The listing builds one solid part. Answer for the finished solid, in the listing's coordinates (mm). Face numbers are marked on the shaded views. A direction names the side the tool comes from. Round coordinates to 2 decimals unless told otherwise and drop trailing zeros. Write each loop counter-clockwise with the first axis right and the second up, starting at its lowest first coordinate (ties: lowest second). Pieces come first, ordered by that corner, then holes. Notation, with made-up numbers: (28.5, -34.5) -> (56.5, -34.5) arc R17 cw to (56.5, -24.5) -> close; hole circle Ø2 at (1.5, 58.25). An arc over 180 degrees is marked (long way). Write each question's results on one line, items separated by ' | '. Start each with the question number.
```python
from build123d import *

# Parameters (mm, degrees)
F0_W     = 342.899989
F0_H     = 117.098217
F0_R     = 2.45745
F1_DEPTH = 19.05


with BuildPart() as f1:
    # F0 (on Top) → F1 (new body)
    with BuildSketch(Plane.XY):
        with Locations((199.415946, 93.865183)):
            Rectangle(F0_W, F0_H)
        with Locations((40.665952, 44.841074)):
            Circle(F0_R, mode=Mode.SUBTRACT)
        with Locations((120.040969, 57.604564)):
            Circle(F0_R, mode=Mode.SUBTRACT)
        with Locations((50.190963, 76.591074)):
            Circle(F0_R, mode=Mode.SUBTRACT)
        with Locations((149.674294, 76.591074)):
            Circle(F0_R, mode=Mode.SUBTRACT)
        with Locations((199.41597, 41.793069)):
            Circle(F0_R, mode=Mode.SUBTRACT)
        with Locations((278.79097, 57.604569)):
            Circle(F0_R, mode=Mode.SUBTRACT)
        with Locations((358.165952, 44.841074)):
            Circle(F0_R, mode=Mode.SUBTRACT)
        with Locations((249.157646, 76.591074)):
            Circle(F0_R, mode=Mode.SUBTRACT)
        with Locations((348.640962, 76.591074)):
            Circle(F0_R, mode=Mode.SUBTRACT)
        with Locations((50.190963, 105.166074)):
            Circle(F0_R, mode=Mode.SUBTRACT)
        with Locations((50.190963, 133.741074)):
            Circle(F0_R, mode=Mode.SUBTRACT)
        with Locations((34.315952, 146.064291)):
            Circle(F0_R, mode=Mode.SUBTRACT)
        with Locations((149.674294, 133.741081)):
            Circle(F0_R, mode=Mode.SUBTRACT)
        with BuildLine():
            ThreePointArc((66.451155, 86.116074), (59.715963, 86.116074), (59.715963, 92.851266))
            Line((59.715963, 92.851266), (59.715963, 117.480882))
            ThreePointArc((59.715963, 117.480882), (59.715963, 124.216074), (66.451155, 124.216074))
            Line((66.451155, 124.216074), (332.380771, 124.216074))
            ThreePointArc((332.380771, 124.216074), (339.115963, 124.216074), (339.115963, 117.480882))
            Line((339.115963, 117.480882), (339.115963, 92.851266))
            ThreePointArc((339.115963, 92.851266), (339.115963, 86.116074), (332.380771, 86.116074))
            Line((332.380771, 86.116074), (66.451155, 86.116074))
        make_face(mode=Mode.SUBTRACT)
        with Locations((348.640962, 105.166074)):
            Circle(F0_R, mode=Mode.SUBTRACT)
        with Locations((249.157646, 133.741081)):
            Circle(F0_R, mode=Mode.SUBTRACT)
        with Locations((199.415967, 147.734329)):
            Circle(F0_R, mode=Mode.SUBTRACT)
        with Locations((348.640962, 133.741074)):
            Circle(F0_R, mode=Mode.SUBTRACT)
        with Locations((364.515952, 146.064291)):
            Circle(F0_R, mode=Mode.SUBTRACT)
    extrude(amount=F1_DEPTH)


solid = f1.part
```
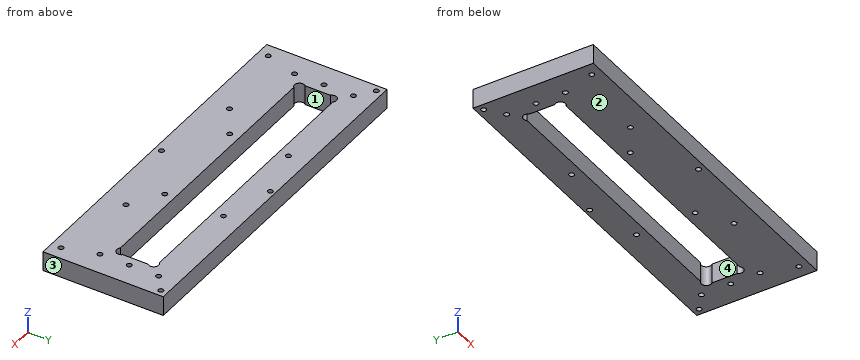
Q1. For the marked faces 1 and 2, determine the directions among +Z, -Z, +X, -X, +Y, -Y from which every point of the face is accessible in a straight line to the end or side of a thin tool.
Q2. Determine the mould class of the marked faces 3 and 4 for opening direction Y: pulls with the +Y half, pulls with the -Y half, needs draft (parallel to the pull), parting line crosses it, or undercut.
Q3. The part is cut by section A-A, the plane x = 258. Write down the section's boundary in (y, z), then the cut area to 3 significant figures.
Q4. The part is cut by section B-B, the plane z = 15.75. State how many separate pieces and enclosed holes the cut face has, then the cut area to 3 significant figures.
Q5. Find the intervals of material crossed by line 1 (Y direction, x = 199, z = 10.25); line 2 (Y direction, x = 303, z = 12.5); line 3 (X direction, y = 98, z = 12.25), in increasing order.
Answers follow:
1) face 1: +Z, -Z | face 2: -Z, +X, -X, +Y, -Y
2) face 3: needs draft | face 4: undercut
3) outline: (35.32, 0) -> (86.12, 0) -> (86.12, 19.05) -> (35.32, 19.05) -> close; (124.22, 0) -> (152.41, 0) -> (152.41, 19.05) -> (124.22, 19.05) -> close | area: 1,500 mm^2
4) separate pieces: 1 | enclosed holes: 19 | area: 29,100 mm^2
5) line 1: 35.32 to 39.37, 44.22 to 86.12, 124.22 to 145.31, 150.16 to 152.41 | line 2: 35.32 to 86.12, 124.22 to 152.41 | line 3: 27.97 to 59.72, 339.12 to 370.87
